Source: CAD feature listing. Evaluate the final solid. Frame: model axes, mm. A direction names the side the tool comes from. Give positions to 0.01 mm unless a question says otherwise; leave off trailing zeros. Order: outer loops, then holes, each group sorted by start corner. A loop starts at its lowest first (then second) coordinate and runs counter-clockwise, first axis right, second up.
1) Section D-D, the plane z = -9. Return loops of the section in (x, y), plus the area to 3 significant figures.
2) First-contact query: P1, Ø1.5, axis at x = 30, z = -1, coming from the +Y side; P2, Ø3, axis at x = 34.5, y = 12, coming from the -Z side; P3, Ø10, axis at x = 27.5, z = -21.5, coming from the +Y side. Flat tips, straight axial feed; report the tip coordinate or a pass-through.
3) Section A-A, the plane y = 6.75. Return loops of the section in (x, z), plus the area to 3 significant figures.
4) Access query for faces 4 (the face through (2, 14.23, -20)), 5 (the face through (22, 9.25, -49)), 6 (the face through (20, 6, -47)). Directions: +Z, -Z, +X, -X, +Y, -Y. A direction counts if a zero-diameter tool reaches every point of the face in a straight line with its end or side. Return the directions, or none.
5) Section C-C, the plane x = 18.5. Return loops of the section in (y, z), plus the area to 3 significant figures.
6) Section B-B, the plane y = 12.25. Return loops of the section in (x, z), plus the area to 4 significant figures.
7) Draft query along X for faces 1 (the face through (0, 7, -25)), 2 (the face through (7, 12, -49)), 3 (the face through (19, 5, -50)). Return one class per face: released by +X, released by -X, zero draft, split by the parting line, or undercut.
8) Material intervals for line 1 (Z direction, x = 23.5, y = 7.25); line 2 (X direction, y = 2.5, z = -28.5); line 3 (Y direction, x = 8.5, z = -25.5), sorted ascending.
```python
from build123d import *

# Parameters (mm, degrees)
SKETCH1_W           = 39.5
SKETCH1_H           = 50
BOSS_EXTRUDE1_DEPTH = 1.5
SKETCH3_W           = 39.5
SKETCH3_H           = 50
SKETCH3_W_2         = 33.5
SKETCH3_H_2         = 44
BOSS_EXTRUDE2_DEPTH = 12.73
SKETCH6_W           = 10
SKETCH6_H           = 5
CUT_EXTRUDE2_DEPTH  = 11.2
SKETCH7_W           = 29.5
SKETCH7_H           = 4.98
CUT_EXTRUDE3_DEPTH  = 3.3


with BuildPart() as part:
    # Sketch1 → Boss-Extrude1 (new body)
    with BuildSketch(Plane(origin=(0, 0, 0), x_dir=(1, 0, 0), z_dir=(0, 1, 0))):
        with Locations((19.75, 25)):
            Rectangle(SKETCH1_W, SKETCH1_H)
    extrude(amount=BOSS_EXTRUDE1_DEPTH)

    # Sketch3 → Boss-Extrude2 (add)
    with BuildSketch(Plane(origin=(0, 1.5, 0), x_dir=(1, 0, 0), z_dir=(0, 1, 0))):
        with Locations((19.75, 25)):
            Rectangle(SKETCH3_W, SKETCH3_H)
        with Locations((19.75, 25)):
            Rectangle(SKETCH3_W_2, SKETCH3_H_2, mode=Mode.SUBTRACT)
    extrude(amount=BOSS_EXTRUDE2_DEPTH)

    # Sketch6 → Cut-Extrude2 (cut)
    with BuildSketch(Plane.XY):
        with Locations((31.5, 11.73)):
            Rectangle(SKETCH6_W, SKETCH6_H)
    extrude(amount=-CUT_EXTRUDE2_DEPTH, mode=Mode.SUBTRACT)

    # Sketch7 → Cut-Extrude3 (cut)
    with BuildSketch(Plane(origin=(0, 0, -50), x_dir=(-1, 0, 0), z_dir=(0, 0, -1))):
        with Locations((-21.75, 11.74)):
            Rectangle(SKETCH7_W, SKETCH7_H)
    extrude(amount=-CUT_EXTRUDE3_DEPTH, mode=Mode.SUBTRACT)


solid = part.part
```
From the geometry:
1. outline: (0, 0) - (39.5, 0) - (39.5, 14.23) - (36.5, 14.23) - (36.5, 1.5) - (3, 1.5) - (3, 14.23) - (0, 14.23) - close
1. area: 136 mm2
2. P1: stops at y = 9.23
2. P2: passes through
2. P3: stops at y = 1.5
3. outline: (0, -50) - (39.5, -50) - (39.5, 0) - (0, 0) - close; hole (3, -47) - (36.5, -47) - (36.5, -3) - (3, -3) - close
3. area: 501 mm2
4. face 4: +Z, -Z, +X, -X, +Y
4. face 5: -Z, +Y
4. face 6: +Y
5. outline: (0, -50) - (9.25, -50) - (9.25, -47) - (1.5, -47) - (1.5, -3) - (14.23, -3) - (14.23, 0) - (0, 0) - close
5. area: 136 mm2
6. outline: (0, -50) - (7, -50) - (7, -47) - (3, -47) - (3, -3) - (26.5, -3) - (26.5, 0) - (0, 0) - close; (36.5, -50) - (39.5, -50) - (39.5, 0) - (36.5, 0) - close
6. area: 382.5 mm2
7. face 1: released by -X
7. face 2: undercut
7. face 3: zero draft
8. line 1: z = -50 to -47, -3 to 0
8. line 2: x = 0 to 3, 36.5 to 39.5
8. line 3: y = 0 to 1.5
